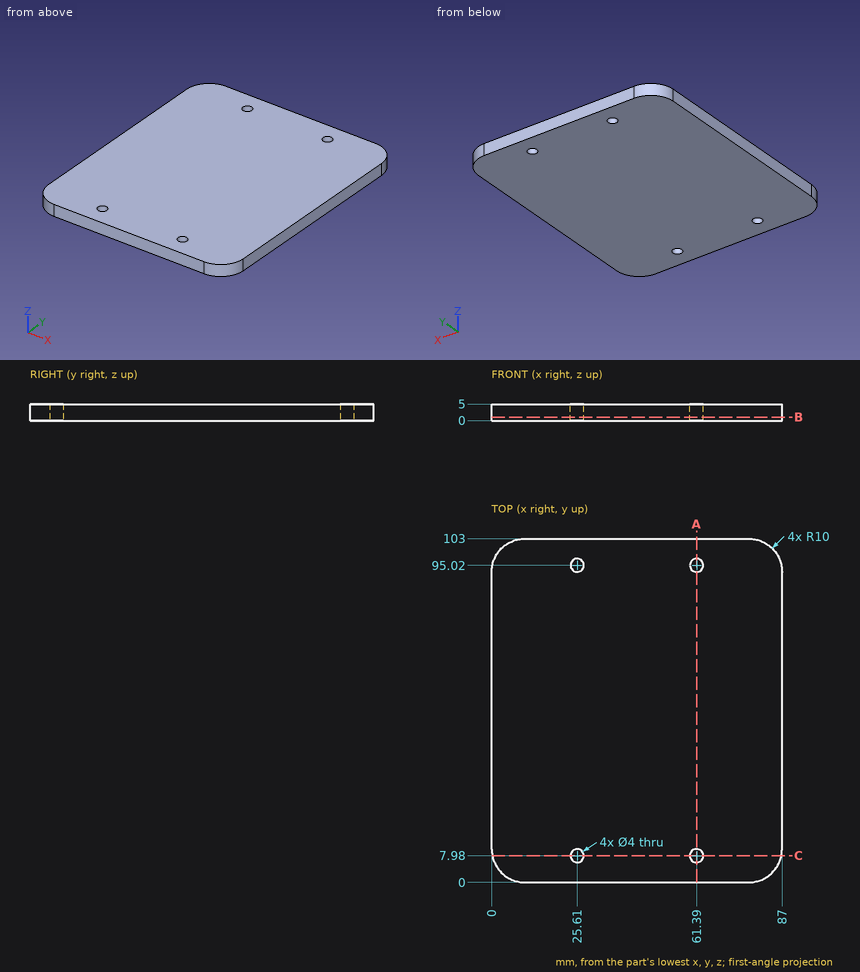
Here's the drawing with two shaded views (mm, measured from the low corner). I have some questions. Coordinates: 2 decimals unless noted, no trailing zeros. Loops run counter-clockwise (first coordinate to the right, second up) from the corner with the lowest first, then second, coordinate; pieces in that order, holes last. Notation, with made-up numbers: (28.5, 81) -> (84.5, 81) arc R30 cw to (84.5, 117) -> close; hole circle Ø4 at (0, 45.5). An arc over 180 degrees is marked (long way). Answer in a Markdown table with one row per item.
(1) Will these pins go through, and if not, where does the flat tip stop? pin 1 Ø5 at (x, y) = (61.39, 7.98) entering from +Z; pin 2 Ø3 at (x, y) = (25.61, 95.02) entering from +Z (3 decimals).
Results found:
| item | result |
|---|---|
| pin 1 | stops at z = 5 |
| pin 2 | passes through |
(2) Imagine slicing it at C-C (y = 7.98). List the corners of the cut face in (x, z) for me, plus the area to 3 significant figures.
Results found:
| item | result |
|---|---|
| outline | (0.21, 0) -> (23.61, 0) -> (23.61, 5) -> (0.21, 5) -> close; (27.61, 0) -> (59.39, 0) -> (59.39, 5) -> (27.61, 5) -> close; (63.39, 0) -> (86.79, 0) -> (86.79, 5) -> (63.39, 5) -> close |
| area | 393 mm^2 |
(3) If I drill on probe 1 along Y at (x, z) = (25.61, 1.8); probe 2 along X at (y, z) = (95, 2.9); probe 3 along Y at (x, z) = (26, 3.75), over which ranges is the centre line in solid material (lowest first)?
Results found:
| item | result |
|---|---|
| probe 1 | y = 0 to 5.98, 9.98 to 93.02, 97.02 to 103 |
| probe 2 | x = 0.2 to 23.61, 27.61 to 59.39, 63.39 to 86.8 |
| probe 3 | y = 0 to 6.02, 9.94 to 93.06, 96.98 to 103 |
(4) Imagine slicing it at B-B (z = 1.05). List the corners of the cut face in (x, y) for me.
Results found:
| item | result |
|---|---|
| outline | (0, 10) arc R10 ccw to (10, 0) -> (77, 0) arc R10 ccw to (87, 10) -> (87, 93) arc R10 ccw to (77, 103) -> (10, 103) arc R10 ccw to (0, 93) -> close; hole circle Ø4 at (25.61, 7.98); hole circle Ø4 at (25.61, 95.02); hole circle Ø4 at (61.39, 7.98); hole circle Ø4 at (61.39, 95.02) |
(5) Imagine slicing it at A-A (x = 61.39). List the corners of the cut face in (y, z) for me, plus the area to 3 significant figures.
Results found:
| item | result |
|---|---|
| outline | (0, 0) -> (5.98, 0) -> (5.98, 5) -> (0, 5) -> close; (9.98, 0) -> (93.02, 0) -> (93.02, 5) -> (9.98, 5) -> close; (97.02, 0) -> (103, 0) -> (103, 5) -> (97.02, 5) -> close |
| area | 475 mm^2 |
